Input: dimensioned drawing with shaded views. Units: mm. Origin: part minimum x, y, z. Round coordinates to 2 decimals unless told otherwise and drop trailing zeros. Order: outer loops, then holes, each group sorted by start corner. A loop starts at its lowest first (then second) coordinate and runs counter-clockwise, first axis right, second up. Notation, with made-up numbers: (-30, 88) - (-19, 88) arc R12 cw to (-19, 101) - close; hole circle Ø9 at (-22.5, 80). An arc over 180 degrees is marked (long way). Return JSON: item names as keys, results as strings. Group by question number.
1) Ray query, line 1 (X direction, y = 38, z = 0.2) (1 decimal); line 2 (Y direction, x = 3.5, z = 1.6) (1 decimal); line 3 (Y direction, x = 31, z = 1.5) (1 decimal). Return the intervals inside material, ascending. Write a range as from..to.
2) Section D-D, the plane x = 4.5. Return loops of the section in (y, z).
3) Section B-B, the plane z = 0.3. Give the number of separate pieces and of enclosed holes in the cut face, plus the area to 3 significant figures.
4) Section A-A, the plane x = 31. Return loops of the section in (y, z).
5) Contact query for flat-ended pins moving along their axis: P1, Ø1.9, axis at x = 4, y = 4, coming from the +Z side; P2, Ø3, axis at x = 30, y = 36, coming from the -Z side. Output: stop coordinate, or through.
6) Section C-C, the plane y = 18. Return loops of the section in (x, z).
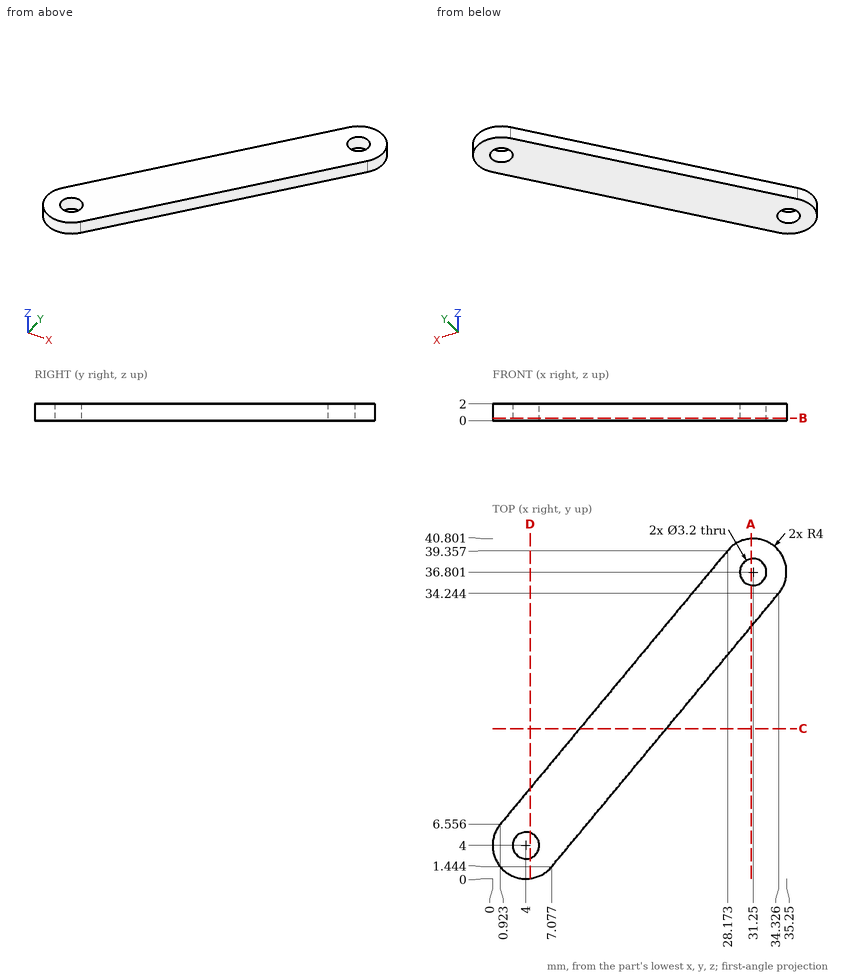
Geometry check:
{
 "1": {"line 1": "27..30.2, 32.3..35.1", "line 2": "0..2.5, 5.5..9.7", "line 3": "30.2..35.2, 38.4..40.8"},
 "2": {"outline": "(0.03, 0) - (2.48, 0) - (2.48, 2) - (0.03, 2) - close; (5.52, 0) - (10.86, 0) - (10.86, 2) - (5.52, 2) - close"},
 "3": {"separate pieces": "1", "enclosed holes": "2", "area": "375 mm2"},
 "4": {"outline": "(30.24, 0) - (35.22, 0) - (35.22, 2) - (30.24, 2) - close; (38.38, 0) - (40.79, 0) - (40.79, 2) - (38.38, 2) - close"},
 "5": {"P1": "through", "P2": "z = 0"},
 "6": {"outline": "(10.43, 0) - (20.83, 0) - (20.83, 2) - (10.43, 2) - close"}
}
